For this review, take the finished solid that the model builds, in its own axes (mm). Face numbers are marked on the shaded views. A direction names the side the tool comes from. Give positions to 0.01 mm unless a question says otherwise; leave off trailing zeros. Order: outer loops, then holes, each group sorted by start corner. A loop starts at its lowest first (then second) coordinate and runs counter-clockwise, first axis right, second up.
Item 1: Consider section B-B (z = -2.25). Give the boundary of the cut face in (x, y), plus the area to 3 significant figures.
Item 2: Consider section D-D (y = 0). Give the boundary of the cut face in (x, z).
Item 3: For P1, Ø6.5, axis at y = -19.5, z = 3.5, coming from the +X side, flat-tipped, find the tip position at first contact; note if it passes through.
Item 4: Consider section C-C (y = 26). Give the boundary of the cut face in (x, z).
Item 5: Consider section A-A (x = 12). Give the boundary of the cut face in (y, z).
Item 6: For probe 1 along Y at (x, z) = (22, 6); probe 2 along Y at (x, z) = (-0.5, -7.75); probe 3 along X at (y, z) = (-36.5, -9.5), list the stretches that pass through material, from the lowest coordinate up.
Item 7: Machinability: for the marked faces 4 and 5, which of the approach directions +Z, -Z, +X, -X, +Y, -Y give a long, thin tool a straight path to every point of the face, cutting with its end or side? Answer none if there is none.
Item 8: The part is to be moulded in two halves that separate along Y. For the marked faces 1, 2 and 3, say which applies: released by +Y, released by -Y, zero draft, split by the parting line, or undercut.
```python
from build123d import *

# Parameters (mm, degrees)
F0_W     = 70
F0_H     = 28
F1_DEPTH = 100
F2_W     = 70
F2_H     = 70
F3_DEPTH = 28.001
F4_R     = 14
F5_DEPTH = 28.001
F6_R     = 5
F7_R     = 1


with BuildPart() as f1:
    # F0 (on Front) → F1 (new body, symmetric)
    with BuildSketch(Plane.XZ):
        Rectangle(F0_W, F0_H)
    extrude(amount=F1_DEPTH, both=True)

    # F2 (on face) → F3 (cut, through all)
    with BuildSketch(Plane.XY.offset(14)):
        with Locations((35, 0)):
            Rectangle(F2_W, F2_H)
    extrude(amount=-F3_DEPTH, mode=Mode.SUBTRACT)

    # F4 (on face) → F5 (cut, through all)
    with BuildSketch(Plane.XY.offset(14)):
        Circle(F4_R)
    extrude(amount=-F5_DEPTH, mode=Mode.SUBTRACT)

    # F6
    f6_edges = [f1.edges().sort_by_distance(p)[0] for p in [
        (-35, 0, 14),
        (35, 67.5, 14),
        (0, 100, 14),
        (0, -100, 14),
        (35, 67.5, -14),
        (-35, 0, -14),
        (35, -67.5, -14),
        (0, -100, -14),
        (0, 100, -14),
    ]]
    fillet(f6_edges, radius=F6_R)

    # F7
    f7_edges = [f1.edges().sort_by_distance(p)[0] for p in [
        (-14, 0, 14),
        (-14, 0, -14),
    ]]
    fillet(f7_edges, radius=F7_R)


solid = f1.part
```
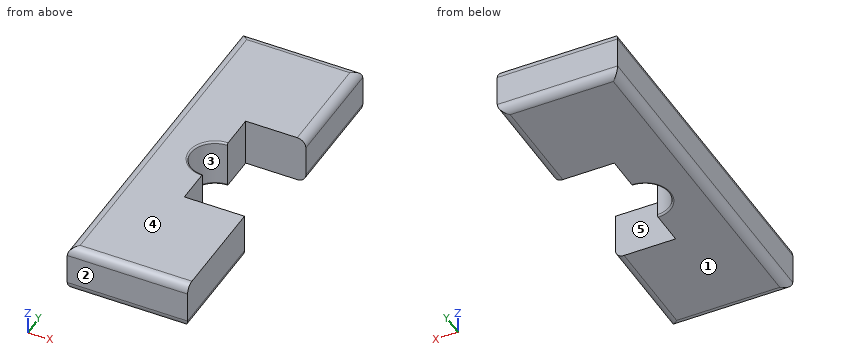
Resolved:
1. outline: (-35, -100) - (35, -100) - (35, -35) - (0, -35) - (0, -14) arc R14 cw to (0, 14) - (0, 35) - (35, 35) - (35, 100) - (-35, 100) - close
1. area: 11,200 mm2
2. outline: (-35, -9) arc R5 ccw to (-30, -14) - (-15, -14) arc R1 ccw to (-14, -13) - (-14, 13) arc R1 ccw to (-15, 14) - (-30, 14) arc R5 ccw to (-35, 9) - close
3. P1: stops at x = 0
4. outline: (-35, -9) arc R5 ccw to (-30, -14) - (0, -14) - (0, 14) - (-30, 14) arc R5 ccw to (-35, 9) - close
5. outline: (-100, -9) arc R5 ccw to (-95, -14) - (-35, -14) - (-35, 14) - (-95, 14) arc R5 ccw to (-100, 9) - close; (35, -14) - (95, -14) arc R5 ccw to (100, -9) - (100, 9) arc R5 ccw to (95, 14) - (35, 14) - close
6. probe 1: y = -100 to -35, 35 to 100
6. probe 2: y = -100 to -13.99, 13.99 to 100
6. probe 3: x = -34.97 to 34.97
7. face 4: +Z, +X, -X, +Y, -Y
7. face 5: +Z, -Z, +X
8. face 1: zero draft
8. face 2: released by -Y
8. face 3: undercut
